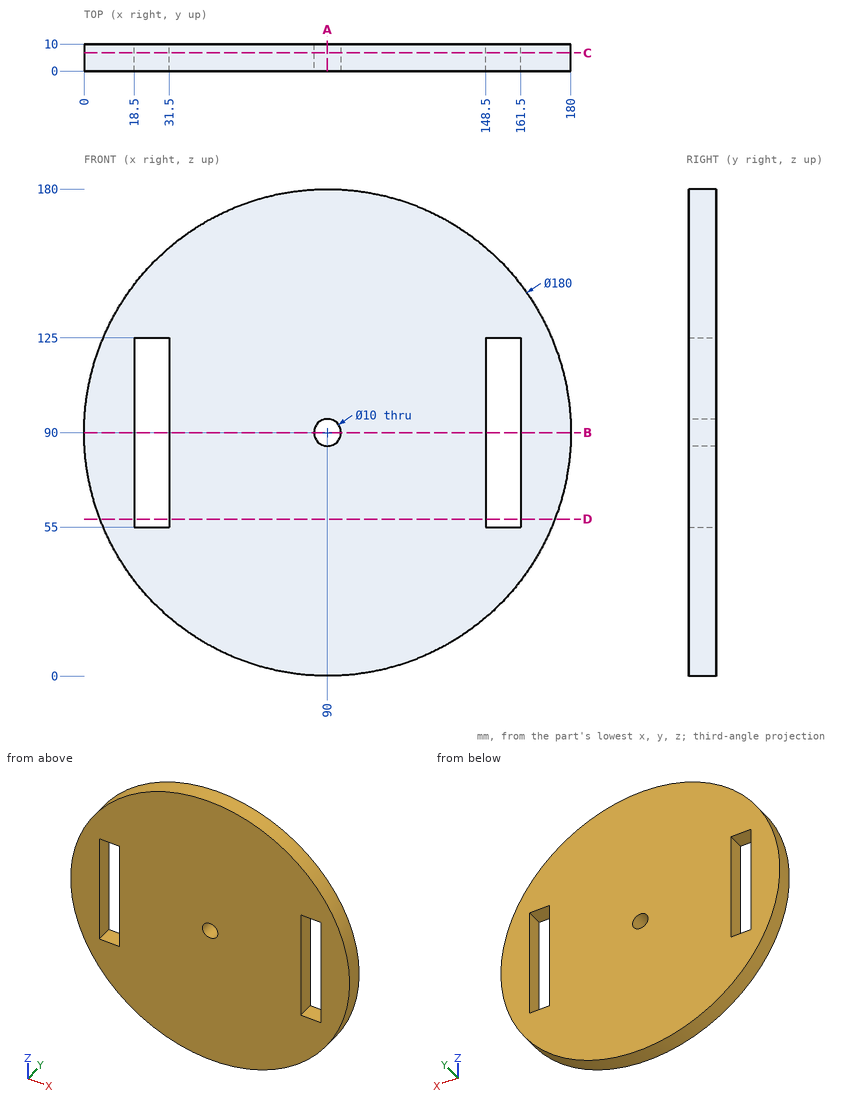
Geometry: see drawing. Coordinates: mm, zero at the bounding-box minimum. Coordinates: 2 decimals unless noted, no trailing zeros. Loops run counter-clockwise (first coordinate to the right, second up) from the corner with the lowest first, then second, coordinate; pieces in that order, holes last. Notation, with made-up numbers: M 75,77 L 134,77 A16 ccw 134,98 Z; hole C 43.25,24 d5. An arc over 180 degrees is marked long. Answer in a Markdown table with one row per item.
Q1. Section C-C on y = 6.75. Return the cut outline in (x, z), plus the area to 3 significant figures.
Answers below:
| item | result |
|---|---|
| outline | C 90,90 d180; hole M 18.5,55 L 31.5,55 L 31.5,125 L 18.5,125 Z; hole C 90,90 d10; hole M 148.5,55 L 161.5,55 L 161.5,125 L 148.5,125 Z |
| area | 23,500 mm^2 |
Q2. Ray query, probe 1 along Z at (x, y) = (90, 4); probe 2 along X at (y, z) = (1, 103); probe 3 along X at (y, z) = (2.5, 113). Return the intervals inside material, ascending. Write a range as from..to.
Answers below:
| item | result |
|---|---|
| probe 1 | z = 0..85, 95..180 |
| probe 2 | x = 0.94..18.5, 31.5..148.5, 161.5..179.06 |
| probe 3 | x = 2.99..18.5, 31.5..148.5, 161.5..177.01 |
Q3. First-contact query: pin 1 (3 mm diameter, centred on x = 158.5, y = 8, fed in from -Z); pin 2 (2 mm diameter, centred on y = 5.5, z = 37, fed in from -X); pin 3 (3 mm diameter, centred on x = 26.5, y = 7, fed in from -Z). Flat tips, straight axial feed; report the tip coordinate or a pass-through.
Answers below:
| item | result |
|---|---|
| pin 1 | stops at z = 29.91 |
| pin 2 | stops at x = 16.54 |
| pin 3 | stops at z = 24.76 |
Q4. Section B-B on z = 90. Return the cut outline in (x, y), plus the area to 3 significant figures.
Answers below:
| item | result |
|---|---|
| outline | M 0,0 L 18.5,0 L 18.5,10 L 0,10 Z; M 31.5,0 L 85,0 L 85,10 L 31.5,10 Z; M 95,0 L 148.5,0 L 148.5,10 L 95,10 Z; M 161.5,0 L 180,0 L 180,10 L 161.5,10 Z |
| area | 1,440 mm^2 |
Q5. Section D-D on z = 58. Return the cut outline in (x, y), plus the area to 3 significant figures.
Answers below:
| item | result |
|---|---|
| outline | M 5.88,0 L 18.5,0 L 18.5,10 L 5.88,10 Z; M 31.5,0 L 148.5,0 L 148.5,10 L 31.5,10 Z; M 161.5,0 L 174.12,0 L 174.12,10 L 161.5,10 Z |
| area | 1,420 mm^2 |
Q6. Section A-A on x = 90. Return the cut outline in (y, z).
Answers below:
| item | result |
|---|---|
| outline | M 0,0 L 10,0 L 10,85 L 0,85 Z; M 0,95 L 10,95 L 10,180 L 0,180 Z |
